Source: CAD feature listing. Evaluate the final solid. Frame: model axes, mm. A direction names the side the tool comes from. Coordinates: 2 decimals unless noted, no trailing zeros. Order: outer loops, then holes, each group sorted by start corner. A loop starts at its lowest first (then second) coordinate and runs counter-clockwise, first axis right, second up. Notation, with made-up numbers: (85, 42) -> (134, 42) arc R16 cw to (134, 57) -> close; hole circle Ø1 at (14, 44.5). An arc over 180 degrees is marked (long way). Write item = value, one per line. Start each with the question number.
Item 1: Set-up query: faces 4 (the cylindrical face through (35.89, 2.01, -1.38)), 5 (the flat face through (33.5, -1.03, 29.68)), 6 (the flat face through (21.2, -15, 16)). Return all of +Z, -Z, +X, -X, +Y, -Y with unobstructed straight access to the full face (end or side cutting, diameter ignored); none if empty.
Item 2: Ray query, line 1 along Z through (x, y) = (15.5, 0.8); line 2 along X through (y, z) = (1.8, 15.5); line 3 along Z through (x, y) = (35.5, 1.65). Return the intervals inside material, ascending. Write a range as [from, to].
Item 3: Section query B-B (x = 0). Output: boundary loops of the cut face in (y, z).
Item 4: Mould query, pull axis X, two halves, no side actions, for faces 1 (the flat face through (-21.2, 1, 16)), 2 (the cylindrical face through (31.851, -12.323, -15.752)), 3 (the cylindrical face through (12.68, -4.5, 24.63)). Classes: released by +X, released by -X, zero draft, split by the parting line, or undercut.
Item 5: Contact query for flat-ended pins moving along their axis: pin 1 (3.5 mm diameter, centred on y = -11.5, z = -18, fed in from -X); pin 2 (7.5 mm diameter, centred on x = 31.5, y = -15, fed in from +Z); pin 3 (2.5 mm diameter, centred on x = -16.5, z = 32, fed in from -Y). Output: stop coordinate, or through.
Item 6: Section query A-A (z = -15.5). Output: boundary loops of the cut face in (x, y), then the cut area to 3 significant figures.
Item 7: Section query C-C (z = 12.5). Output: boundary loops of the cut face in (x, y).
Item 8: Section query D-D (x = 15.5). Output: boundary loops of the cut face in (y, z), then the cut area to 3 significant figures.
Autodesk Inventor part; units mm, degrees
ref_plane "YZ Plane" through (0, 0, 0) normal (1, 0, 0) x (0, 1, 0)
ref_plane "XZ Plane" through (0, 0, 0) normal (0, 1, 0) x (-1, 0, 0)
ref_plane "XY Plane" through (0, 0, 0) normal (0, 0, 1) x (1, 0, 0)
sketch "Boceto1" plane through (0, 0, 0) normal (0, 1, 0) x (-1, 0, 0)
  line L0 (-21.2, 21.2) -> (21.2, 21.2)
  line L1 (21.2, 21.2) -> (21.2, -21.2)
  line L2 (21.2, -21.2) -> (-21.2, -21.2)
  line L3 (-21.2, -21.2) -> (-21.2, 21.2)
  line L4 (-21.2, 21.2) -> (21.2, -21.2) construction
  line L5 (21.2, 21.2) -> (-21.2, -21.2) construction
  circle A0 centre (0, 0) radius 11.2
  point P0 (0, 0)
  dimension "d0" = 42.4
  dimension "d1" = 42.4
  dimension "d2" = 22.4
extrude "Extrusión1" add sketch "Boceto1" along normal blind 3
sketch "Boceto2" plane through (0, 3, 0) normal (0, 1, 0) x (1, 0, 0)
  circle A0 centre (-15.5, -15.5) radius 1.7
  line L0 (15.5, -15.5) -> (-15.5, -15.5)
  line L1 (-15.5, -15.5) -> (-15.5, 15.5)
  line L2 (-15.5, 15.5) -> (15.5, 15.5)
  line L3 (15.5, 15.5) -> (15.5, -15.5)
  line L4 (15.5, -15.5) -> (-15.5, 15.5) construction
  line L5 (-15.5, -15.5) -> (15.5, 15.5) construction
  point P0 (0, 0)
  dimension "d5" = 31
  dimension "d6" = 31
  dimension "d7" = 3.4
extrude "Extrusión2" cut sketch "Boceto2" against normal through all contours L0 L1 A0 | A0 L1 L0
pattern_circular "Patrón circular1" count 4 over 360 about axis through (0, 0, 0) along (0, 1, 0) of "Extrusión2"
sketch "Boceto13" plane through (0, 3, 0) normal (0, 1, 0) x (1, 0, 0)
  line L0 (-21.2, -21.2) -> (21.2, -21.2)
  line L1 (21.2, -21.2) -> (41.5, -21.2)
  line L2 (41.5, -21.2) -> (41.5, 21.2)
  line L3 (41.5, 21.2) -> (21.2, 21.2)
  line L4 (21.2, 21.2) -> (21.2, -21.2)
  line L5 (21.2, 21.2) -> (-21.2, 21.2)
  line L6 (41.5, -10.15) -> (21.2, -10.15)
  line L7 (21.2, -10.15) -> (21.2, 10.15)
  line L8 (21.2, 10.15) -> (41.5, 10.15)
  line L9 (41.5, 10.15) -> (41.5, -10.15)
  line L10 (41.5, -10.15) -> (21.2, 10.15) construction
  line L11 (21.2, -10.15) -> (41.5, 10.15) construction
  circle A0 centre (31.5, 0) radius 2.7
  point P0 (0, 0)
  point P1 (31.35, 0)
  dimension "d43" = 20.3
  dimension "d44" = 20.3
  dimension "d45" = 20.3
  dimension "d61" = 5.4
  dimension "d62" = 10
extrude "Extrusión8" add sketch "Boceto13" against normal blind 33
sketch "Boceto14" plane through (0, -30, 0) normal (0, -1, 0) x (1, 0, 0)
  line L0 (21.2, 21.2) -> (21.2, -21.2)
  line L1 (41.5, -10.15) -> (21.2, -10.15)
  line L2 (21.2, -10.15) -> (21.2, 10.15)
  line L3 (21.2, 10.15) -> (41.5, 10.15)
  line L4 (41.5, 10.15) -> (41.5, -10.15)
  line L5 (41.5, -10.15) -> (21.2, 10.15) construction
  line L6 (21.2, -10.15) -> (41.5, 10.15) construction
  point P0 (0, 0)
  point P1 (31.35, 0)
  dimension "d49" = 20.3
extrude "Extrusión9" cut sketch "Boceto14" against normal up to surface (30 mm away)
sketch "Boceto15" plane through (-21.2, 0, -21.2) normal (0, 0, -1) x (-1, 0, 0)
  line L0 (-42.4, 0) -> (0, 0)
  line L1 (0, 0) -> (0, 3)
  line L2 (-62.7, 3) -> (0, 3)
  line L3 (-62.7, 3) -> (-62.7, -30)
  line L4 (-42.4, -30) -> (-62.7, -30)
  line L5 (-42.4, 0) -> (-42.4, -30)
  line L6 (0, 0) -> (0, 3)
  line L7 (-42.4, -30) -> (-62.7, -30)
  line L8 (0, 0) -> (-42.4, -30)
  point P0 (-21.2, 0)
extrude "Extrusión10" add sketch "Boceto15" along normal blind 2
mirror "Simetría1" about plane through (0, 0, 0) normal (0, 0, 1) of "Extrusión10"
sketch "Boceto16" plane through (-21.2, 0, -23.2) normal (0, 0, -1) x (-1, 0, 0)
  circle A0 centre (-52.7, -15) radius 2.7
  line L0 (-62.7, 3) -> (-62.7, -30)
  line L1 (-62.7, -30) -> (-42.4, -30)
  point P0 (-21.2, 0)
  dimension "d54" = 10
  dimension "d55" = 5.4
  dimension "d57" = 15
extrude "Extrusión11" cut sketch "Boceto16" against normal through all
fillet "Empalme1" radius 2 2 edges at (41.5, -30, -16.675) (41.5, -30, 16.675)
sketch "Boceto17" plane through (-21.2, 0, -23.2) normal (0, 0, -1) x (-1, 0, 0)
  circle A0 centre (-52.7, -15) radius 2.7
  circle A1 centre (-52.7, -15) radius 4.65
  point P0 (-21.2, 0)
  dimension "d63" = 9.3
extrude "Extrusión12" cut sketch "Boceto17" against normal blind 2 contours A0 | A1
sketch "Boceto18" plane through (0, 3, 0) normal (0, 1, 0) x (1, 0, 0)
  circle A0 centre (31.5, 0) radius 2.7
  circle A1 centre (31.5, 0) radius 4.6
  point P0 (0, 0)
  dimension "d66" = 9.2
extrude "Extrusión13" cut sketch "Boceto18" against normal blind 2 contours A0 | A1
mirror "Simetría2" about plane through (0, 0, 0) normal (0, 0, 1) of "Extrusión12"
sketch "Boceto19" plane through (0, 3, 0) normal (0, 1, 0) x (1, 0, 0)
  line L0 (21.2, -21.2) -> (-21.2, -21.2)
  line L1 (-21.2, 21.2) -> (-21.2, -21.2)
  line L2 (-21.2, -21.2) -> (41.5, -21.2)
  line L3 (41.5, -21.2) -> (41.5, -43.2)
  line L4 (41.5, -43.2) -> (-21.2, -43.2)
  line L5 (-21.2, -43.2) -> (-21.2, -21.2)
  line L6 (-21.2, -23.2) -> (41.5, -23.2)
  line L7 (41.5, -23.2) -> (41.5, 23.2)
  point P0 (0, 0)
  dimension "d69" = 20
extrude "Extrusión14" add sketch "Boceto19" against normal blind 6
sketch "Boceto20" plane through (0, -3, 0) normal (0, -1, 0) x (1, 0, 0)
  circle A0 centre (-15.2, 33.2) radius 2.7
  circle A1 centre (35.5, 33.2) radius 2.7
  line L0 (-21.2, 43.2) -> (-21.2, 21.2)
  line L1 (41.5, 23.2) -> (41.5, 43.2)
  line L2 (41.5, 43.2) -> (-21.2, 43.2)
  point P0 (0, 0)
  dimension "d72" = 5.4
  dimension "d73" = 6
  dimension "d74" = 6
  dimension "d75" = 10
  dimension "d76" = 10
extrude "Extrusión15" cut sketch "Boceto20" against normal through all
sketch "Boceto21" plane through (0, -3, 0) normal (0, -1, 0) x (1, 0, 0)
  circle A0 centre (-15.2, 33.2) radius 2.7
  circle A1 centre (-15.2, 33.2) radius 4.05
  circle A2 centre (35.5, 33.2) radius 2.7
  circle A3 centre (35.5, 33.2) radius 4.05
  line L0 (35.5, 37.8765) -> (39.55, 35.5383)
  line L1 (39.55, 35.5383) -> (39.55, 30.8617)
  line L2 (39.55, 30.8617) -> (35.5, 28.5235)
  line L3 (35.5, 28.5235) -> (31.45, 30.8617)
  line L4 (31.45, 30.8617) -> (31.45, 35.5383)
  line L5 (31.45, 35.5383) -> (35.5, 37.8765)
  line L6 (-15.2, 37.8765) -> (-11.15, 35.5383)
  line L7 (-11.15, 35.5383) -> (-11.15, 30.8617)
  line L8 (-11.15, 30.8617) -> (-15.2, 28.5235)
  line L9 (-15.2, 28.5235) -> (-19.25, 30.8617)
  line L10 (-19.25, 30.8617) -> (-19.25, 35.5383)
  line L11 (-19.25, 35.5383) -> (-15.2, 37.8765)
  point P0 (0, 0)
  dimension "d79" = 8.1
extrude "Extrusión16" cut sketch "Boceto21" against normal blind 4 contours A0 | A1 | L7 L8 A1 | A1 L6 L7 | A1 L11 L6 | L8 L9 A1 | A1 L10 L11 | L9 L10 A1 | A2 | A3 | L1 L2 A3 | A3 L0 L1 | A3 L5 L0 | L2 L3 A3 | A3 L4 L5 | L3 L4 A3
fillet "Empalme2" radius 3 2 edges at (-21.2, 0, 43.2) (41.5, 0, 43.2)
fillet "Empalme3" radius 5 1 edges at (12.27, -3, 23.2)
sketch "Boceto7" plane through (21.2, 0, -21.2) normal (0, 0, -1) x (-1, 0, 0)
  line L0 (42.4, 0) -> (42.4, 3)
  line L1 (42.4, 3) -> (-20.3, 3)
  line L2 (-20.3, 3) -> (-20.3, -27)
  line L3 (-20.3, -27) -> (42.4, -27)
  line L4 (42.4, -27) -> (42.4, 3)
  line L5 (0, 0) -> (0, 3)
  point P0 (21.2, 0)
  point P1 (35.6, 0)
  dimension "d23" = 20.3
  dimension "d24" = 30
sketch "Boceto8" plane through (0, 3, 0) normal (0, 1, 0) x (1, 0, 0)
  line L0 (17.8, 17.8) -> (-17.8, 17.8)
  line L1 (17.8, -17.8) -> (16.8, -17.8)
  line L2 (16.8, -17.8) -> (16.8, 17.8)
  line L3 (16.8, 17.8) -> (17.8, 17.8)
  line L4 (17.8, 17.8) -> (17.8, -17.8)
  point P0 (0, 0)
  dimension "d27" = 1
sketch "Boceto9" plane through (17.8, 0, -21.8) normal (0, 0, -1) x (-1, 0, 0)
  circle A0 centre (-10.3, -4.5) radius 2.7
  circle A1 centre (-10.3, -19.5) radius 2.7
  line L0 (-20.3, 3) -> (-20.3, -27)
  line L1 (35.6, 3) -> (-20.3, 3)
  line L2 (-20.3, -27) -> (35.6, -27)
  point P0 (17.8, 0)
  dimension "d30" = 5.4
  dimension "d31" = 10
  dimension "d32" = 7.5
  dimension "d33" = 7.5
  dimension "d41" = 80
  dimension "d42" = 20.3
sketch "Boceto10" plane through (17.8, 0, -17.8) normal (0, 0, 1) x (1, 0, 0)
  line L0 (20.3, 3) -> (20.3, -27)
  line L1 (-1, 3) -> (20.3, 3)
  line L2 (20.3, -27) -> (0.3, -27)
  line L3 (0.3, -27) -> (0.3, 3)
  line L4 (0.3, 3) -> (20.3, 3)
  line L5 (20.3, 3) -> (20.3, -27)
  circle A0 centre (10.3, -4.5) radius 2.7
  circle A1 centre (10.3, -19.5) radius 2.7
  line L6 (-1, 0) -> (-35.6, 0)
  line L7 (-35.6, -27) -> (-35.6, 0)
  line L8 (20.3, -27) -> (-35.6, -27)
  line L9 (20.3, 3) -> (20.3, -27)
  line L10 (-1, 3) -> (20.3, 3)
  line L11 (-1, 3) -> (-1, 0)
  point P0 (-17.8, 0)
  dimension "d36" = 20
sketch "Boceto3" plane through (-21.2, 0, 21.2) normal (0, 0, 1) x (1, 0, 0)
  line L0 (0, 0) -> (0, 3)
  line L1 (0, 3) -> (62.7, 3)
  line L2 (62.7, 3) -> (62.7, -30)
  line L3 (62.7, -30) -> (0, -30)
  line L4 (0, -30) -> (0, 3)
  line L5 (42.4, 0) -> (42.4, 3)
  line L6 (0, 0) -> (42.4, 0)
  point P0 (21.2, 0)
  dimension "d13" = 20.3
  dimension "d14" = 30
  dimension "d17" = 5.4
  dimension "d18" = 10
  dimension "d19" = 7.5
  dimension "d20" = 7.5
  dimension "d21" = 20.3
  dimension "d22" = 20.3
properties part number "NEMA14 support"
Computed:
q1.face_4 = +Y
q1.face_5 = -Y
q1.face_6 = -X, -Y
q2.line_1 = [-23.2, -17.2], [-13.8, 13.8], [17.2, 43.2]
q2.line_2 = [-21.2, -17.2], [-13.8, 13.8], [17.2, 41.5]
q2.line_3 = [-23.2, -2.27], [2.27, 30.5], [35.9, 43.2]
q3.outline = (-15, -23.2) -> (3, -23.2) -> (3, -11.2) -> (0, -11.2) -> (0, -21.2) -> (-15, -21.2) -> close; (-15, 21.2) -> (0, 21.2) -> (0, 11.2) -> (3, 11.2) -> (3, 43.2) -> (-3, 43.2) -> (-3, 28.2) arc R5 cw to (-8, 23.2) -> (-15, 23.2) -> close
q4.face_1 = released by -X
q4.face_2 = undercut
q4.face_3 = zero draft
q5.pin_1 = 21.2
q5.pin_2 = 21.2
q5.pin_3 = 1
q6.outline = (-21.2, 0) -> (-17.2, 0) -> (-17.2, 3) -> (-21.2, 3) -> close; (-13.8, 0) -> (13.8, 0) -> (13.8, 3) -> (-13.8, 3) -> close; (17.2, 0) -> (21.2, 0) -> (21.2, -30) -> (39.5, -30) arc R2 ccw to (41.5, -28) -> (41.5, 3) -> (17.2, 3) -> close; hole circle Ø5.4 at (31.5, -15)
q6.area = 753 mm^2
q7.outline = (-21.2, 0) -> (21.2, 0) -> (21.2, -30) -> (39.5, -30) arc R2 ccw to (41.5, -28) -> (41.5, 3) -> (-21.2, 3) -> close; hole circle Ø5.4 at (31.5, -15)
q8.outline = (-25.97, -23.2) -> (3, -23.2) -> (3, -17.2) -> (0, -17.2) -> (0, -21.2) -> (-25.97, -21.2) -> close; (-25.97, 21.2) -> (0, 21.2) -> (0, 17.2) -> (3, 17.2) -> (3, 43.2) -> (-3, 43.2) -> (-3, 28.2) arc R5 cw to (-8, 23.2) -> (-25.97, 23.2) -> close; (0, -13.8) -> (3, -13.8) -> (3, 13.8) -> (0, 13.8) -> close
q8.area = 348 mm^2
